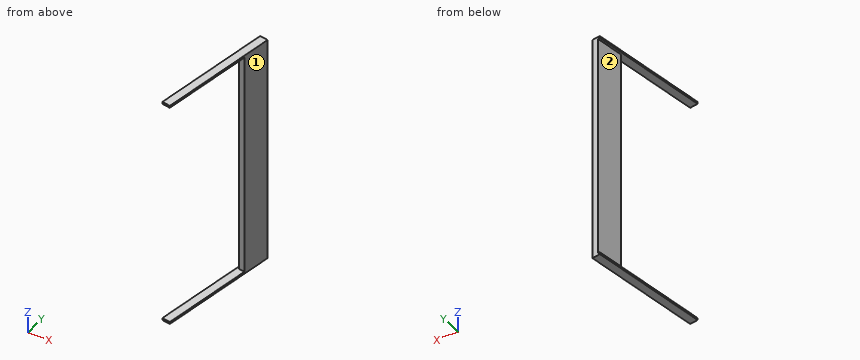
Autodesk Inventor part; units mm, degrees
ref_plane "YZ Plane" through (0, 0, 0) normal (1, 0, 0) x (0, 1, 0)
ref_plane "XZ Plane" through (0, 0, 0) normal (0, 1, 0) x (-1, 0, 0)
ref_plane "XY Plane" through (0, 0, 0) normal (0, 0, 1) x (1, 0, 0)
sketch "Sketch1" plane through (0, 0, 0) normal (0, 0, 1) x (1, 0, 0)
  line L0 (0, 0) -> (112.2718, 740.8411)
  line L1 (50.2265, -7.6116) -> (162.4983, 733.2294)
  line L2 (162.4983, 733.2294) -> (112.2718, 740.8411)
  line L3 (50.2265, -7.6116) -> (0, 0)
  line L4 (162.4983, 733.2294) -> (135.8576, 557.4366)
  line L5 (135.8576, 557.4366) -> (98.1877, 563.1454)
  line L6 (98.1877, 563.1454) -> (124.8285, 738.9382)
  line L7 (124.8285, 738.9382) -> (162.4983, 733.2294)
  dimension "d0" = 749.3
  dimension "d2" = 50.8
  dimension "d3" = 177.8
  dimension "d4" = 38.1
extrude "Extrusion1" add sketch "Sketch1" along normal blind 1384.3 contours L2 L1 L5 L6
extrude "Extrusion2" add sketch "Sketch1" along normal blind 12.7 contours L0 L2 L6 L5 L1 L3
sketch "Sketch2" plane through (0, 0, 1384.3) normal (0, 0, 1) x (1, 0, 0)
  line L0 (162.4983, 733.2294) -> (124.8285, 738.9382)
  line L1 (162.4983, 733.2294) -> (112.2718, 740.8411)
  line L2 (0, 0) -> (50.2265, -7.6116)
  line L3 (112.2718, 740.8411) -> (0, 0)
  line L4 (50.2265, -7.6116) -> (162.4983, 733.2294)
  line L5 (0, 0) -> (50.2265, -7.6116)
  line L6 (50.2265, -7.6116) -> (162.4983, 733.2294)
  line L7 (135.8576, 557.4366) -> (162.4983, 733.2294)
  line L8 (112.2718, 740.8411) -> (162.4983, 733.2294)
  line L9 (162.4983, 733.2294) -> (50.2265, -7.6116)
  dimension "d9" = 50.8
extrude "Extrusion3" add sketch "Sketch2" against normal blind 12.7
properties part number "BackRest"
CAD build for the part. Positions are in the model's coordinates, mm. Face numbers are marked on the shaded views. Coordinates: 2 decimals unless noted, no trailing zeros. Order: outer loops, then holes, each group sorted by start corner. A loop starts at its lowest first (then second) coordinate and runs counter-clockwise, first axis right, second up.
(1) Drill centre lines: L1, parallel to Z at x = 90, y = 572.5; L2, parallel to Y at x = 131, z = 984; L3, parallel to X at y = 602.5, z = 118.5. Where is each one in solid material? Low to high.
Solution:
L1: z = 0 to 12.7, 1371.6 to 1384.3
L2: y = 558.17 to 738
L3: x = 104.15 to 142.69
(2) Saw through at B-B, the plane y = 473.5. Write the cut outline in (x, z), and give its area (3 significant figures).
Solution:
outline: (71.76, 0) - (123.14, 0) - (123.14, 12.7) - (71.76, 12.7) - close; (71.76, 1371.6) - (123.14, 1371.6) - (123.14, 1384.3) - (71.76, 1384.3) - close
area: 1,310 mm2
(3) Pin check, flat tips, straight feed: pin 1 Ø3 at (y, z) = (612, 412.5) entering from +X; pin 2 Ø10 at (x, y) = (59.5, 329) entering from -Z; pin 3 Ø12 at (x, y) = (118, 367) entering from +Z. Stop position of each tip, or through.
Solution:
pin 1: stops at x = 144.35
pin 2: stops at z = 0
pin 3: passes through
(4) Mould opens along Z. For the marked faces 1 and 2 say: released by +Z, released by -Z, zero draft, split by the parting line, or undercut.
Solution:
face 1: zero draft
face 2: undercut
(5) Saw through at D-D, the plane z = 1116. Write the cut outline in (x, y).
Solution:
outline: (98.19, 563.15) - (135.86, 557.44) - (162.5, 733.23) - (124.83, 738.94) - close
(6) Saw through at A-A, the plane x = 81. Write the cut outline in (y, z), and give its area (3 significant figures).
Solution:
outline: (195.45, 0) - (534.49, 0) - (534.49, 12.7) - (195.45, 12.7) - close; (195.45, 1371.6) - (534.49, 1371.6) - (534.49, 1384.3) - (195.45, 1384.3) - close
area: 8,610 mm2
(7) Saw through at C-C, the plane y = 635. Write the cut outline in (x, z).
Solution:
outline: (96.23, 0) - (147.61, 0) - (147.61, 1384.3) - (96.23, 1384.3) - (96.23, 1371.6) - (109.08, 1371.6) - (109.08, 12.7) - (96.23, 12.7) - close
